Here's how the part is built. I have some questions about the finished solid (model axes, mm). A direction names the side the tool comes from. Round coordinates to 2 decimals unless told otherwise and drop trailing zeros. Order: outer loops, then holes, each group sorted by start corner. A loop starts at its lowest first (then second) coordinate and runs counter-clockwise, first axis right, second up. Notation, with made-up numbers: (50.25, 32) - (81.25, 32) arc R16 ccw to (81.25, 47) - close; hole circle Ø2 at (18.5, 20.5). An arc over 180 degrees is marked (long way). Answer as a JSON object with one key per item and string values.
```python
from build123d import *

# Parameters (mm, degrees)
F0_W      = 101.6
F0_H      = 103.766376869
F1_DEPTH  = 25.4
F2_DEPTH  = 6.35
F3_R      = 5.08
F4_W      = 88.9
F4_H      = 4.550592151
F5_DEPTH  = 25.4
F6_W      = 41.91
F6_H      = 35.5364200096
F6_W_2    = 5.08
F7_DEPTH  = 12.7
F8_W      = 88.9
F8_H      = 6.35
F9_DEPTH  = 12.7
F11_DEPTH = 25.4


with BuildPart() as f1:
    # F0 (on Front) → F1 (new body)
    with BuildSketch(Plane.XZ):
        with Locations((-0.5670151889, -2.7032315751)):
            Rectangle(F0_W, F0_H)
        Polygon((-45.0170151889, 3.280592151), (-45.0170151889, 42.8299568594), (-6.9170151889, 42.8299568594), align=None, mode=Mode.SUBTRACT)
        Polygon((-3.1070151889, 3.280592151), (-41.2070151889, 3.280592151), (-3.1070151889, 42.8299568594), align=None, mode=Mode.SUBTRACT)
        Polygon((1.9729848111, 42.8299568594), (40.0729848111, 3.280592151), (1.9729848111, 3.280592151), align=None, mode=Mode.SUBTRACT)
        Polygon((5.7829848111, 42.8299568594), (43.8829848111, 42.8299568594), (43.8829848111, 3.280592151), align=None, mode=Mode.SUBTRACT)
    extrude(amount=F1_DEPTH)

    # F0 (on Front) → F2 (join)
    with BuildSketch(Plane.XZ):
        Polygon((-6.9170151889, 42.8299568594), (-45.0170151889, 42.8299568594), (-45.0170151889, 3.280592151), align=None)
        Polygon((-3.1070151889, 42.8299568594), (-41.2070151889, 3.280592151), (-3.1070151889, 3.280592151), align=None)
        Polygon((1.9729848111, 3.280592151), (40.0729848111, 3.280592151), (1.9729848111, 42.8299568594), align=None)
        Polygon((43.8829848111, 3.280592151), (43.8829848111, 42.8299568594), (5.7829848111, 42.8299568594), align=None)
    extrude(amount=F2_DEPTH)

    # F3
    f3_edges = [f1.edges().sort_by_distance(p)[0] for p in [
        (-51.367015, -12.7, 49.179957),
        (50.232985, -12.7, 49.179957),
    ]]
    fillet(f3_edges, radius=F3_R)

    # F4 (on face) → F5 (cut)
    with BuildSketch(Plane.XZ.offset(25.4)):
        with Locations((-0.5670151889, -4.0747039245)):
            Rectangle(F4_W, F4_H)
    extrude(amount=-F5_DEPTH, mode=Mode.SUBTRACT)

    # F6 (on face) → F7 (cut)
    with BuildSketch(Plane.XZ.offset(25.4)):
        with Locations((-24.0620151889, -30.4682100048)):
            Rectangle(F6_W, F6_H)
        with Locations((22.9279848111, -30.4682100048)):
            Rectangle(F6_W, F6_H)
        with Locations((-0.5670151889, -30.4682100048)):
            Rectangle(F6_W_2, F6_H)
    extrude(amount=-F7_DEPTH, mode=Mode.SUBTRACT)

    # F8 (on face) → F9 (cut)
    with BuildSketch(Plane.XZ.offset(25.4)):
        with Locations((-0.5670151889, -51.4114200096)):
            Rectangle(F8_W, F8_H)
    extrude(amount=-F9_DEPTH, mode=Mode.SUBTRACT)

    # F10 (on face) → F11 (cut)
    with BuildSketch(Plane.XZ.offset(25.4)):
        with BuildLine():
            ThreePointArc((-28.5070151889, -4.0747039245), (-32.3170151889, -0.2647039245), (-36.1270151889, -4.0747039245))
            Line((-36.1270151889, -4.0747039245), (-28.5070151889, -4.0747039245))
        make_face()
        with BuildLine():
            ThreePointArc((34.9929848111, -4.0747039245), (31.1829848111, -0.2647039245), (27.3729848111, -4.0747039245))
            Line((27.3729848111, -4.0747039245), (34.9929848111, -4.0747039245))
        make_face()
        with BuildLine():
            Line((34.9929848111, -4.0747039245), (27.3729848111, -4.0747039245))
            ThreePointArc((27.3729848111, -4.0747039245), (31.1829848111, -7.8847039245), (34.9929848111, -4.0747039245))
        make_face()
        with BuildLine():
            ThreePointArc((18.4829848111, -4.0747039245), (14.6729848111, -0.2647039245), (10.8629848111, -4.0747039245))
            Line((10.8629848111, -4.0747039245), (18.4829848111, -4.0747039245))
        make_face()
        with BuildLine():
            Line((18.4829848111, -4.0747039245), (10.8629848111, -4.0747039245))
            ThreePointArc((10.8629848111, -4.0747039245), (14.6729848111, -7.8847039245), (18.4829848111, -4.0747039245))
        make_face()
        with BuildLine():
            ThreePointArc((4.5129848111, -4.0747039245), (-0.5670151889, 1.0052960755), (-5.6470151889, -4.0747039245))
            Line((-5.6470151889, -4.0747039245), (4.5129848111, -4.0747039245))
        make_face()
        with BuildLine():
            Line((4.5129848111, -4.0747039245), (-5.6470151889, -4.0747039245))
            ThreePointArc((-5.6470151889, -4.0747039245), (-0.5670151889, -9.1547039245), (4.5129848111, -4.0747039245))
        make_face()
        with BuildLine():
            ThreePointArc((-11.9970151889, -4.0747039245), (-15.8070151889, -0.2647039245), (-19.6170151889, -4.0747039245))
            Line((-19.6170151889, -4.0747039245), (-11.9970151889, -4.0747039245))
        make_face()
        with BuildLine():
            Line((-11.9970151889, -4.0747039245), (-19.6170151889, -4.0747039245))
            ThreePointArc((-19.6170151889, -4.0747039245), (-15.8070151889, -7.8847039245), (-11.9970151889, -4.0747039245))
        make_face()
        with BuildLine():
            Line((-28.5070151889, -4.0747039245), (-36.1270151889, -4.0747039245))
            ThreePointArc((-36.1270151889, -4.0747039245), (-32.3170151889, -7.8847039245), (-28.5070151889, -4.0747039245))
        make_face()
    extrude(amount=-F11_DEPTH, mode=Mode.SUBTRACT)


solid = f1.part
```
1. Imagine slicing it at C-C (y = -18.25). Give the number of separate pieces and of enclosed holes in the cut face, plus the area to 3 significant figures.
Responses:
{"separate pieces": "1", "enclosed holes": "5", "area": "3,300 mm2"}
2. Imagine slicing it at D-D (x = -27). List the corners of the cut face in (y, z) for me, plus the area to 3 significant figures.
Responses:
{"outline": "(-25.4, -12.7) - (-12.7, -12.7) - (-12.7, -54.59) - (0, -54.59) - (0, -6.35) - (-25.4, -6.35) - close; (-25.4, -1.8) - (0, -1.8) - (0, 49.18) - (-25.4, 49.18) - (-25.4, 42.83) - (-6.35, 42.83) - (-6.35, 21.98) - (-25.4, 21.98) - (-25.4, 18.03) - (-6.35, 18.03) - (-6.35, 3.28) - (-25.4, 3.28) - close", "area": "1,310 mm2"}
3. Imagine slicing it at A-A (z = -4). List the corners of the cut face in (x, y) for me.
Responses:
{"outline": "(-51.37, -25.4) - (-45.02, -25.4) - (-45.02, 0) - (-51.37, 0) - close; (43.88, -25.4) - (50.23, -25.4) - (50.23, 0) - (43.88, 0) - close"}
4. For P1, Ø14, axis at x = 1, y = -17.5, coming from the -Z side; P2, Ø3, axis at x = 37.5, y = -18.5, coming from the -Z side, each with a flat end and sliding along its axis, tell me the tip position at first contact or that it passes through.
Responses:
{"P1": "z = -54.59", "P2": "z = -12.7"}
5. If I drill on L1, parallel to X at y = -15.25, z = -30; L2, parallel to Z at x = 31, y = -9; L3, parallel to X at y = -19.5, z = 9, over which ranges is the centre line in solid material (lowest first)? Write a range as [from, to].
Responses:
{"L1": "[-51.37, -45.02], [43.88, 50.23]", "L2": "[-54.59, -7.88], [-0.27, 3.28], [12.7, 16.65], [42.83, 49.18]", "L3": "[-51.37, -45.02], [-39.51, -35.7], [-3.11, 1.97], [34.56, 38.37], [43.88, 50.23]"}
6. For faces 1 (the face through (-15.757, -12.878, -0.265)), 2 (the face through (-1, -12.7, -33)), 3 (the face through (-22.42, -15.74, 22.78)), 4 (the face through (-1, 0, 10)), which set-ups out of +Z, -Z, +X, -X, +Y, -Y let a thin tool reach every point of the face, with its end or its side?
Responses:
{"face 1": "+Y, -Y", "face 2": "-Z, -Y", "face 3": "-Y", "face 4": "+Z, -Z, +X, -X, +Y"}
7. Thinking about a two-plate mould opening in X: for faces 5 (the face through (-1, -7, -54.586)), 6 (the face through (-49.92, -12.88, 47.65)), 7 (the face through (-22, -16, 3.281)), 8 (the face through (50.233, -13, -6)), which applies, pulls with the +X half, pulls with the -X half, needs draft (parallel to the pull), parting line crosses it, or undercut?
Responses:
{"face 5": "needs draft", "face 6": "pulls with the -X half", "face 7": "undercut", "face 8": "pulls with the +X half"}
8. Imagine slicing it at B-B (x = 13.5). List the corners of the cut face in (y, z) for me.
Responses:
{"outline": "(-25.4, -12.7) - (-12.7, -12.7) - (-12.7, -54.59) - (0, -54.59) - (0, -7.7) - (-25.4, -7.7) - close; (-25.4, -0.45) - (0, -0.45) - (0, 49.18) - (-25.4, 49.18) - (-25.4, 42.83) - (-6.35, 42.83) - (-6.35, 34.82) - (-25.4, 34.82) - (-25.4, 30.86) - (-6.35, 30.86) - (-6.35, 3.28) - (-25.4, 3.28) - close"}
